from build123d import *

# Parameters (mm, degrees)
F0_W         = 127
F0_H         = 76.2
F1_DEPTH     = 25.4
F2_R         = 8.4769821521
F2_R_2       = 9.2372123091
F3_DEPTH     = 25.401
F4_W         = 12.7
F4_H         = 25.4
F6_W         = 25.4
F6_H         = 6.35
F8_W         = 25.4
F8_H         = 6.35
F10_R        = 5.08
F11_T1_DEPTH = 51.5282991577
F11_T3_DEPTH = 153.1282991577


# Not quite as in the source:
# - a fillet or chamfer that OpenCascade refuses, or shapes differently, is made with other operations: its cross-section is extruded or revolved along the edge and cut away or added


with BuildPart() as f1:
    # F0 (on Top) → F1 (new body)
    with BuildSketch(Plane.XY):
        Rectangle(F0_W, F0_H)
    extrude(amount=F1_DEPTH)

    # F2 (on face) → F3 (cut, through all)
    with BuildSketch(Plane.XY.offset(25.4)):
        with Locations((-51.2244440438, 25.4412265494)):
            Circle(F2_R)
        with Locations((-49.6174134314, -21.1683232337)):
            Circle(F2_R)
        with Locations((52.2232688963, 27.0741768181)):
            Circle(F2_R_2)
        with Locations((49.5918877423, -21.6549038887)):
            Circle(F2_R)
    extrude(amount=-F3_DEPTH, mode=Mode.SUBTRACT)

    # F4 (on Front) → F5 (revolve)
    with BuildSketch(Plane.XZ):
        with Locations((6.35, 38.1)):
            Rectangle(F4_W, F4_H)
    revolve(axis=Axis((0, 0, 38.1), (0, 0, 1)))

    # F6 (on Front) → F7 (revolve)
    with BuildSketch(Plane.XZ):
        with Locations((12.7, 53.975)):
            Rectangle(F6_W, F6_H)
    revolve(axis=Axis((0, 0, 53.975), (0, 0, -1)))

    # F8 (on Front) → F9 (revolve)
    with BuildSketch(Plane.XZ):
        with Locations((12.7, 28.575)):
            Rectangle(F8_W, F8_H)
    revolve(axis=Axis((0, 0, 28.575), (0, 0, -1)))

    # F10
    f10_edges = [f1.edges().sort_by_distance(p)[0] for p in [
        (-25.4, 0, 57.15),
        (-25.4, 0, 25.4),
    ]]
    fillet(f10_edges, radius=F10_R)

    # F11: chamfer of 5.08 on 8 edges, made by hand

    # F11_s2 → F11_t1 (cut)
    with BuildSketch(Plane.XY.offset(-13.0641495789)):
        Polygon((-58.42, -38.1), (-63.5, -33.02), (-63.5, -38.1), align=None)
        Polygon((63.5, -33.02), (58.42, -38.1), (63.5, -38.1), align=None)
        Polygon((63.5, 33.02), (58.42, 38.1), (63.5, 38.1), align=None)
        Polygon((-58.42, 38.1), (-63.5, 33.02), (-63.5, 38.1), align=None)
    extrude(amount=F11_T1_DEPTH, mode=Mode.SUBTRACT)

    # F11_s4 → F11_t3 (cut)
    with BuildSketch(Plane.YZ.offset(-76.5641495789)):
        Polygon((-38.1, 5.08), (-33.02, 0), (-38.1, 0), align=None)
        Polygon((-33.02, 25.4), (-38.1, 20.32), (-38.1, 25.4), align=None)
        Polygon((38.1, 5.08), (33.02, 0), (38.1, 0), align=None)
        Polygon((33.02, 25.4), (38.1, 20.32), (38.1, 25.4), align=None)
    extrude(amount=F11_T3_DEPTH, mode=Mode.SUBTRACT)


solid = f1.part
Verification items for the finished model (mm, model axes). A direction names the side the tool comes from. Coordinates: 2 decimals unless noted, no trailing zeros. Write each loop counter-clockwise with the first axis right and the second up, starting at its lowest first coordinate (ties: lowest second). Pieces come first, ordered by that corner, then holes. Notation, with made-up numbers: M 14.25,-24 L 41.25,-24 A14 ccw 41.25,-4 Z; hole C -17,25.5 d5. An arc over 180 degrees is marked long. Use CSV: the item, a comma, the result in double quotes.
Q1. Set-up check for faces 1 (the flat face through (-5, -12, 31.75)), 2 (the flat face through (-1, -38.1, 13)), 3 (the cylindrical face through (-5.506, 24.796, 51.444)): record each of +Z, -Z, +X, -X, +Y, -Y from which the full face is reachable in a straight line by a thin tool's end or side.
Computed values:
face 1,"none"
face 2,"+Z, -Z, +X, -X, -Y"
face 3,"+Z"
Q2. Go/stop test with flat-tipped pins: P1, Ø16.5, axis at x = 52.22, y = 27.07, coming from the +Z side; P2, Ø22, axis at x = -51.22, y = 25.44, coming from the -Z side; P3, Ø5, axis at x = -3, z = 41.5, coming from the +Y side. Record where each tip stops, or that it passes through.
Computed values:
P1,"through"
P2,"z = 0"
P3,"y = 12.69"
Q3. Section check D-D, the plane z = 41.5. Enter the section's corners in (x, y).
Computed values:
outline,"C 0,0 d25.4"
Q4. Section check B-B, the plane x = 0. Enter the section's corners in (y, z).
Computed values:
outline,"M -38.1,5.08 L -33.02,0 L 33.02,0 L 38.1,5.08 L 38.1,20.32 L 33.02,25.4 L 30.48,25.4 A5.08 cw 25.4,30.48 L 25.4,31.75 L 12.7,31.75 L 12.7,50.8 L 25.4,50.8 L 25.4,52.07 A5.08 ccw 20.32,57.15 L -20.32,57.15 A5.08 ccw -25.4,52.07 L -25.4,50.8 L -12.7,50.8 L -12.7,31.75 L -25.4,31.75 L -25.4,30.48 A5.08 cw -30.48,25.4 L -33.02,25.4 L -38.1,20.32 Z"
Q5. Mould release check, pull along Y, two halves, no side actions. Record for faces 4 (the cylindrical face through (42.865, -26.813, 12.878)), 5 (the flat face through (-0.89, -35.52, 22.9)), 6 (the flat face through (-0.89, 35.52, 22.9)): pulls with the +Y half, pulls with the -Y half, needs draft (parallel to the pull), parting line crosses it, or undercut.
Computed values:
face 4,"undercut"
face 5,"pulls with the -Y half"
face 6,"pulls with the +Y half"
Q6. Section check A-A, the plane y = 0. Enter the section's corners in (x, z), and give its area (3 significant figures).
Computed values:
outline,"M -63.5,0 L 63.5,0 L 63.5,25.4 L 30.48,25.4 A5.08 cw 25.4,30.48 L 25.4,31.75 L 12.7,31.75 L 12.7,50.8 L 25.4,50.8 L 25.4,52.07 A5.08 ccw 20.32,57.15 L -20.32,57.15 A5.08 ccw -25.4,52.07 L -25.4,50.8 L -12.7,50.8 L -12.7,31.75 L -25.4,31.75 L -25.4,30.48 A5.08 cw -30.48,25.4 L -63.5,25.4 Z"
area,"4,350 mm²"
Q7. Section check C-C, the plane x = 49.5. Enter the section's corners in (y, z).
Computed values:
outline,"M -38.1,5.08 L -33.02,0 L -30.13,0 L -30.13,25.4 L -33.02,25.4 L -38.1,20.32 Z; M -13.18,0 L 18.25,0 L 18.25,25.4 L -13.18,25.4 Z; M 35.9,2.88 L 38.1,5.08 L 38.1,20.32 L 35.9,22.52 Z"
Q8. Thickness scan on line 1 along X through (y, z) = (33, 21); line 2 along X through (y, z) = (20, 7); line 3 along Z through (x, y) = (9, -17). Record the ranges inside material, lowest first. Write a range as [from, to].
Computed values:
line 1,"[-63.5, -55.06], [-47.39, 45.14], [59.31, 63.5]"
line 2,"[-63.5, -57.72], [-44.72, 46.28], [58.16, 63.5]"
line 3,"[0, 31.75], [50.8, 57.15]"
